from build123d import *

# Parameters (mm, degrees)
SKETCH2_W             = 7
SKETCH2_H             = 30
BOSS_EXTRUDE1_DEPTH   = 25
SKETCH5_R             = 6.5
CUT_EXTRUDE1_DEPTH    = 7
M5X0_8_TAPPED_HOLE2_D = 4.2


with BuildPart() as part:
    # Sketch2 → Boss-Extrude1 (new body)
    with BuildSketch(Plane(origin=(0, 0, 0), x_dir=(1, 0, 0), z_dir=(0, 1, 0))):
        Rectangle(SKETCH2_W, SKETCH2_H)
    extrude(amount=BOSS_EXTRUDE1_DEPTH)

    # Sketch5 → Cut-Extrude1 (cut)
    with BuildSketch(Plane(origin=(3.5, 0, 0), x_dir=(0, 0, -1), z_dir=(1, 0, 0))):
        with Locations((0, 8.72)):
            Circle(SKETCH5_R)
    extrude(amount=-CUT_EXTRUDE1_DEPTH, mode=Mode.SUBTRACT)

    # M5x0.8 Tapped Hole2 (through all)
    with Locations(Plane(origin=(3.5, 0, 0), x_dir=(0, 0, -1), z_dir=(1, 0, 0))):
        with Locations((10, 20), (-10, 20)):
            Hole(M5X0_8_TAPPED_HOLE2_D / 2)


solid = part.part
Model file for the job. Use its own axes, mm. Give positions to 0.01 mm unless a question says otherwise; leave off trailing zeros. Loops run counter-clockwise (first coordinate to the right, second up) from the corner with the lowest first, then second, coordinate; pieces in that order, holes last. Notation, with made-up numbers: (-17, 85) -> (17, 85) arc R15 cw to (17, 92) -> close; hole circle Ø4 at (23, 21.5). An arc over 180 degrees is marked (long way). Use a Markdown table: item, result. Add a question column.
(1) Slice it at C-C on x = 3. List the corners of the cut face in (y, z).
(2) Wall check: line 1 along Z through (x, y) = (-1.25, 8.5); line 2 along Y through (x, z) = (2.25, 0); line 3 along Y through (x, z) = (-0.25, -10). Give the ranges that are in metal, low to high.
(3) Mould opens along Z. For faces 1 (the cylindrical face through (0.049, 15.165, 0.846)), 2 (the flat face through (-3.5, 15, 4)), 3 (the flat face through (0, 12, -15)) say: +Z half, -Z half, draft (parallel to the pull), parting line (faces both ways), or undercut.
(4) Slice it at D-D on y = 20. List the corners of the cut face in (x, z), and give its area (3 significant figures).
(5) Slice it at B-B on y = 8.72. List the corners of the cut face in (x, z), and give its area (3 significant figures).
(6) Slice it at A-A on z = -10. List the corners of the cut face in (x, y), and give its area (3 significant figures).
Filled sheet:
| question | item | result |
|---|---|---|
| 1 | outline | (0, -15) -> (25, -15) -> (25, 15) -> (0, 15) -> close; hole circle Ø13 at (8.72, 0); hole circle Ø4.2 at (20, -10); hole circle Ø4.2 at (20, 10) |
| 2 | line 1 | -15 to -6.5, 6.5 to 15 |
| 2 | line 2 | 0 to 2.22, 15.22 to 25 |
| 2 | line 3 | 0 to 17.9, 22.1 to 25 |
| 3 | face 1 | undercut |
| 3 | face 2 | draft |
| 3 | face 3 | -Z half |
| 4 | outline | (-3.5, -15) -> (3.5, -15) -> (3.5, -12.1) -> (-3.5, -12.1) -> close; (-3.5, -7.9) -> (3.5, -7.9) -> (3.5, 7.9) -> (-3.5, 7.9) -> close; (-3.5, 12.1) -> (3.5, 12.1) -> (3.5, 15) -> (-3.5, 15) -> close |
| 4 | area | 151 mm2 |
| 5 | outline | (-3.5, -15) -> (3.5, -15) -> (3.5, -6.5) -> (-3.5, -6.5) -> close; (-3.5, 6.5) -> (3.5, 6.5) -> (3.5, 15) -> (-3.5, 15) -> close |
| 5 | area | 119 mm2 |
| 6 | outline | (-3.5, 0) -> (3.5, 0) -> (3.5, 17.9) -> (-3.5, 17.9) -> close; (-3.5, 22.1) -> (3.5, 22.1) -> (3.5, 25) -> (-3.5, 25) -> close |
| 6 | area | 146 mm2 |
